The model under review builds one solid part; all positions refer to its coordinate system, in mm. Face numbers are marked on the shaded views. Round coordinates to 2 decimals unless told otherwise and drop trailing zeros. Order: outer loops, then holes, each group sorted by start corner. A loop starts at its lowest first (then second) coordinate and runs counter-clockwise, first axis right, second up.
1) Clearance check with flat-ended pins moving along their axes: P1, Ø1.6, axis at y = 11.5, z = -3.5, coming from the -X side; P2, Ø4, axis at y = -10, z = -3.5, coming from the +X side; P3, Ø15, axis at x = 87.5, z = -3.5, coming from the -Y side. State where each tip first meets the part, or that it passes through.
2) Mouldability with a two-part tool opening along Z and no side actions: class the marked faces 1, 2 and 3 as pulls with the +Z half, pulls with the -Z half, needs draft (parallel to the pull), parting line crosses it, or undercut.
3) To check wall thickness, follow L1, parallel to Z at x = 81, y = 2; L2, parallel to Y at x = 81, z = -0.25. State the ranges of each line that lie inside material, in increasing order.
4) Consider section C-C (x = 152.5). Give the boundary of the cut face in (y, z) (3 decimals).
5) Consider section B-B (z = -3.5). Give the boundary of the cut face in (x, y).
6) Consider section A-A (x = 19.05). Give the boundary of the cut face in (y, z) (3 decimals).
7) Consider section D-D (x = 87.5). Give the boundary of the cut face in (y, z) (3 decimals).
from build123d import *

# Parameters (mm, degrees)
F1_DEPTH = 184.15
F3_DEPTH = 33.3375
F4_R     = 3.96875
F5_DEPTH = 25.401
F7_DEPTH = 25.401
F9_DEPTH = 25.4010001


with BuildPart() as f1:
    # F0 (on Right) → F1 (new body)
    with BuildSketch(Plane.YZ):
        with BuildLine():
            Line((-9.525, -12.7), (9.525, -12.7))
            ThreePointArc((9.525, -12.7), (11.7700640303, -11.7700640303), (12.7, -9.525))
            Line((12.7, -9.525), (12.7, 9.525))
            ThreePointArc((12.7, 9.525), (11.7700640303, 11.7700640303), (9.525, 12.7))
            Line((9.525, 12.7), (-9.525, 12.7))
            ThreePointArc((-9.525, 12.7), (-11.7700640303, 11.7700640303), (-12.7, 9.525))
            Line((-12.7, 9.525), (-12.7, -9.525))
            ThreePointArc((-12.7, -9.525), (-11.7700640303, -11.7700640303), (-9.525, -12.7))
        make_face()
        with BuildLine():
            Line((-9.525, 10.5918), (9.525, 10.5918))
            ThreePointArc((9.525, 10.5918), (10.2793415142, 10.2793415142), (10.5918, 9.525))
            Line((10.5918, 9.525), (10.5918, -9.525))
            ThreePointArc((10.5918, -9.525), (10.2793415142, -10.2793415142), (9.525, -10.5918))
            Line((9.525, -10.5918), (-9.525, -10.5918))
            ThreePointArc((-9.525, -10.5918), (-10.2793415142, -10.2793415142), (-10.5918, -9.525))
            Line((-10.5918, -9.525), (-10.5918, 9.525))
            ThreePointArc((-10.5918, 9.525), (-10.2793415142, 10.2793415142), (-9.525, 10.5918))
        make_face(mode=Mode.SUBTRACT)
    extrude(amount=F1_DEPTH)

    # F2 (on face) → F3 (cut)
    with BuildSketch(Plane(origin=(0, 0, 0), x_dir=(0, -1, 0), z_dir=(-1, 0, 0))):
        with BuildLine():
            ThreePointArc((-12.7, 9.525), (-12.6535126242, 10.0663259281), (-12.5154118044, 10.5918))
            Line((-12.5154118044, 10.5918), (-16.0259325057, 10.5918))
            Line((-16.0259325057, 10.5918), (-16.0259325057, -10.5918))
            Line((-16.0259325057, -10.5918), (-12.5154118044, -10.5918))
            ThreePointArc((-12.5154118044, -10.5918), (-12.6535126242, -10.0663259281), (-12.7, -9.525))
            Line((-12.7, -9.525), (-12.7, 9.525))
        make_face()
        with BuildLine():
            Line((-7.5196851976, -10.5918), (-7.5196851976, 10.5918))
            Line((-7.5196851976, 10.5918), (-9.525, 10.5918))
            ThreePointArc((-9.525, 10.5918), (-10.2793415142, 10.2793415142), (-10.5918, 9.525))
            Line((-10.5918, 9.525), (-10.5918, -9.525))
            ThreePointArc((-10.5918, -9.525), (-10.2793415142, -10.2793415142), (-9.525, -10.5918))
            Line((-9.525, -10.5918), (-7.5196851976, -10.5918))
        make_face()
        with BuildLine():
            ThreePointArc((-10.5918, 9.525), (-10.2793415142, 10.2793415142), (-9.525, 10.5918))
            Line((-9.525, 10.5918), (-12.5154118044, 10.5918))
            ThreePointArc((-12.5154118044, 10.5918), (-12.6535126242, 10.0663259281), (-12.7, 9.525))
            Line((-12.7, 9.525), (-12.7, -9.525))
            ThreePointArc((-12.7, -9.525), (-12.6535126242, -10.0663259281), (-12.5154118044, -10.5918))
            Line((-12.5154118044, -10.5918), (-9.525, -10.5918))
            ThreePointArc((-9.525, -10.5918), (-10.2793415142, -10.2793415142), (-10.5918, -9.525))
            Line((-10.5918, -9.525), (-10.5918, 9.525))
        make_face()
    extrude(amount=-F3_DEPTH, mode=Mode.SUBTRACT)

    # F4 (on face) → F5 (cut, through all)
    with BuildSketch(Plane.XY.offset(12.7)):
        with Locations((19.05, 0)):
            Circle(F4_R)
    extrude(amount=-F5_DEPTH, mode=Mode.SUBTRACT)

    # F6 (on face) → F7 (cut, through all)
    with BuildSketch(Plane.XY.offset(12.7)):
        with BuildLine():
            ThreePointArc((2.5522160579, 9.525), (4.2134911079, 11.9490796254), (6.2278308065, 14.0888068044))
            Line((6.2278308065, 14.0888068044), (1.4018084571, 20.3806743289))
            ThreePointArc((1.4018084571, 20.3806743289), (-5.47164532, 11.203546833), (-7.9097950815, 0))
            Line((-7.9097950815, 0), (0, 0))
            Line((0, 0), (0, 9.525))
            Line((0, 9.525), (2.5522160579, 9.525))
        make_face()
        with BuildLine():
            ThreePointArc((0, 0), (0.6491130092, 4.9305028092), (2.5522160579, 9.525))
            Line((2.5522160579, 9.525), (0, 9.525))
            Line((0, 9.525), (0, 0))
        make_face()
    extrude(amount=-F7_DEPTH, mode=Mode.SUBTRACT)

    # F8 (on face) → F9 (cut, through all)
    with BuildSketch(Plane.XY.offset(12.7)):
        Polygon((184.15, -9.525), (184.15, 6.35), (54.8585004559, -9.525), align=None)
        Polygon((188.5616199521, -29.5797611986), (184.15, 6.35), (184.15, -9.525), (54.8585004559, -9.525), (47.0669696314, -10.481679691), (51.4785895836, -46.4114408897), align=None)
    extrude(amount=-F9_DEPTH, mode=Mode.SUBTRACT)


solid = f1.part
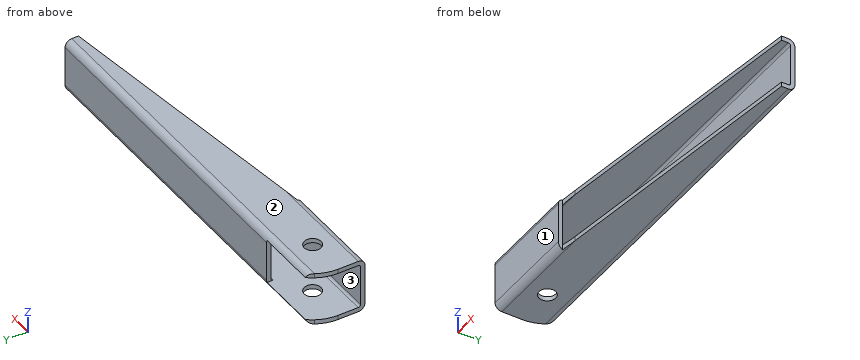
Answer below:
1. P1: stops at x = 33.34
1. P2: stops at x = 47.25
1. P3: stops at y = -5.82
2. face 1: needs draft
2. face 2: pulls with the +Z half
2. face 3: undercut
3. L1: z = -12.7 to -10.59, 10.59 to 12.7
3. L2: y = 10.59 to 12.7
4. outline: (2.464, -12.7) - (9.525, -12.7) arc R3.175 ccw to (12.7, -9.525) - (12.7, 9.525) arc R3.175 ccw to (9.525, 12.7) - (2.464, 12.7) - (2.464, 10.592) - (9.525, 10.592) arc R1.067 cw to (10.592, 9.525) - (10.592, -9.525) arc R1.067 cw to (9.525, -10.592) - (2.464, -10.592) - close
5. outline: (0, -12.7) - (47.34, -12.7) - (47.08, -10.59) - (0, -10.59) - close; (33.34, 10.59) - (184.15, 10.59) - (184.15, 12.7) - (33.34, 12.7) - close
6. outline: (-12.7, -9.525) arc R3.175 ccw to (-9.525, -12.7) - (-3.969, -12.7) - (-3.969, -10.592) - (-9.525, -10.592) arc R1.067 cw to (-10.592, -9.525) - (-10.592, 9.525) arc R1.067 cw to (-9.525, 10.592) - (-3.969, 10.592) - (-3.969, 12.7) - (-9.525, 12.7) arc R3.175 ccw to (-12.7, 9.525) - close; (3.969, -12.7) - (9.525, -12.7) arc R3.175 ccw to (12.515, -10.592) - (3.969, -10.592) - close; (3.969, 10.592) - (12.515, 10.592) arc R3.175 ccw to (9.525, 12.7) - (3.969, 12.7) - close
7. outline: (-5.517, -12.7) - (9.525, -12.7) arc R3.175 ccw to (12.7, -9.525) - (12.7, 9.525) arc R3.175 ccw to (9.525, 12.7) - (-5.517, 12.7) - (-5.517, 10.592) - (9.525, 10.592) arc R1.067 cw to (10.592, 9.525) - (10.592, -9.525) arc R1.067 cw to (9.525, -10.592) - (-5.517, -10.592) - close
